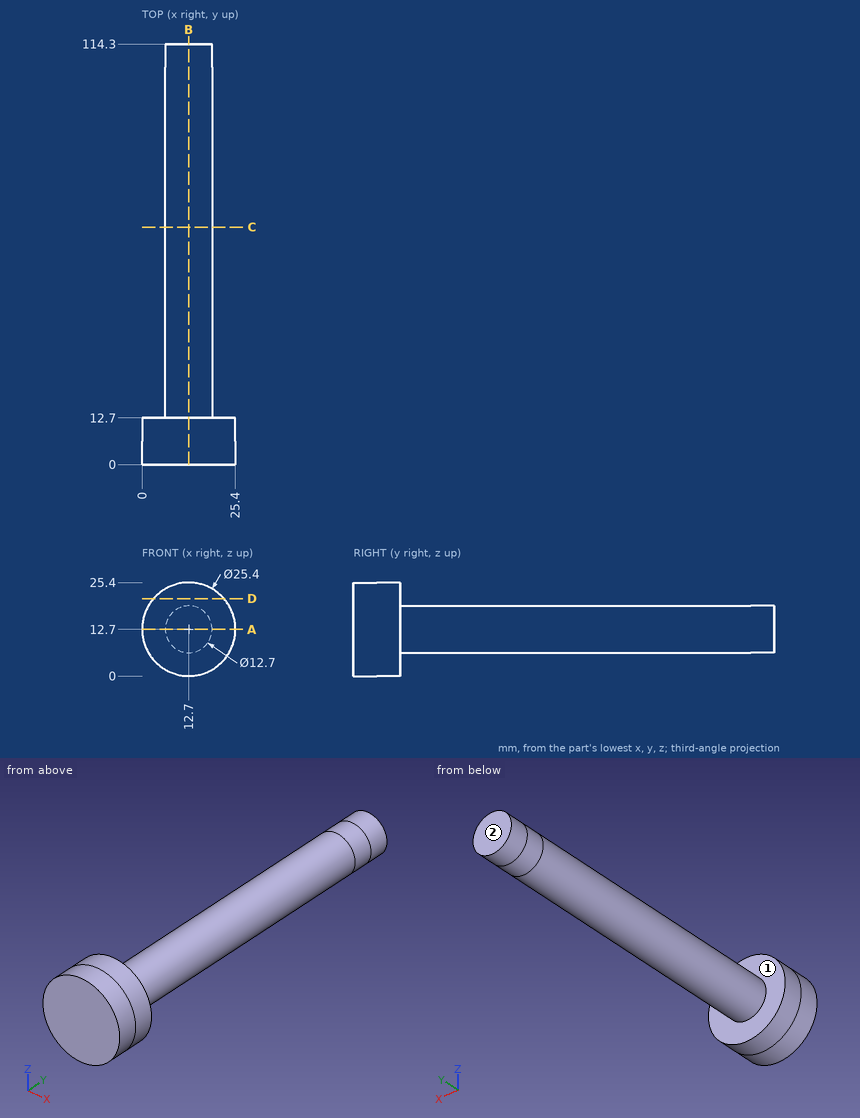
Design review of the part shown in the three views and the two pictorial views. Dimensions are in mm from the part's minimum x, y and z. A direction names the side the tool comes from. Round coordinates to 2 decimals unless told otherwise and drop trailing zeros. Write each loop counter-clockwise with the first axis right and the second up, starting at its lowest first coordinate (ties: lowest second). Pieces come first, ordered by that corner, then holes. Notation, with made-up numbers: M -11.75,35.25 L 23.25,35.25 A21 ccw 23.25,46.25 Z; hole C 83.25,-29.5 d6. An arc over 180 degrees is marked long. Use a Markdown table: item, result. Add a question column.
Q1. We need section C-C, the plane y = 64.5. State the section outline as (x, z) points, plus the area to 3 significant figures.
Q2. Machinability: for the marked faces 1 and 2, which of the approach directions +Z, -Z, +X, -X, +Y, -Y give a long, thin tool a straight path to every point of the face, cutting with its end or side? Answer none if there is none.
Q3. We need section A-A, the plane z = 12.7. State the section outline as (x, y) points, plus the area to 3 significant figures.
Q4. We need section B-B, the plane x = 12.7. State the section outline as (y, z) points.
Q5. Insertion check: pin 1 (3 mm diameter, centred on x = 8, y = 84.5, fed in from -Z); pin 2 (1.5 mm diameter, centred on x = 10, y = 47, fed in from +Z); pin 3 (6 mm diameter, centred on x = 5, y = 80.5, fed in from -Z). Each pin has a flat end and moves straight along its axis. Give the tip position at first contact, or say it passes through.
Q6. To check wall thickness, follow line 1 (Y direction, x = 5, z = 21.5); line 2 (Z direction, x = 13, y = 56.5); line 3 (X direction, y = 104.5, z = 12.75). State the ranges of each line that lie inside material, in increasing order.
Q7. We need section D-D, the plane z = 21. State the section outline as (x, y) points.
Findings below:
| question | item | result |
|---|---|---|
| 1 | outline | C 12.7,12.7 d12.7 |
| 1 | area | 127 mm² |
| 2 | face 1 | +Y |
| 2 | face 2 | +Z, -Z, +X, -X, +Y |
| 3 | outline | M 0,0 L 25.4,0 L 25.4,12.7 L 19.05,12.7 L 19.05,114.3 L 6.35,114.3 L 6.35,12.7 L 0,12.7 Z |
| 3 | area | 1,610 mm² |
| 4 | outline | M 0,0 L 12.7,0 L 12.7,6.35 L 114.3,6.35 L 114.3,19.05 L 12.7,19.05 L 12.7,25.4 L 0,25.4 Z |
| 5 | pin 1 | stops at z = 7.22 |
| 5 | pin 2 | stops at z = 18.74 |
| 5 | pin 3 | stops at z = 8.43 |
| 6 | line 1 | y = 0 to 12.7 |
| 6 | line 2 | z = 6.36 to 19.04 |
| 6 | line 3 | x = 6.35 to 19.05 |
| 7 | outline | M 3.09,0 L 22.31,0 L 22.31,12.7 L 3.09,12.7 Z |
